Geometry: final body of the model. Coordinates: model frame, mm. A direction names the side the tool comes from. Give positions to 0.01 mm unless a question says otherwise; leave off trailing zeros. Write each loop counter-clockwise with the first axis right and the second up, starting at its lowest first coordinate (ties: lowest second). Pieces come first, ordered by that corner, then holes.
Autodesk Inventor part; units mm, degrees
ref_plane "BODY_N_XY" through (84, 0, 0) normal (0, 0, -1) x (1, 0, 0)
ref_plane "BODY_N_YZ" through (84, 0, 0) normal (1, 0, 0) x (0, -1, 0)
ref_plane "BODY_N_ZX" through (84, 0, 0) normal (0, -1, 0) x (0, 0, -1)
sketch "Sketch_8" plane through (0, 0, 0) normal (0, 0, 1) x (1, 0, 0)
  line L0 (0, 0) -> (-8, 0)
  line L1 (-8, 0) -> (-8, 3.3865)
  line L2 (-8, 3.3865) -> (-7.3865, 4)
  line L3 (-7.3865, 4) -> (0, 4)
  line L4 (0, 4) -> (0, 0)
  line L5 (0, 0) -> (-8, 0)
revolve "Revolution1" add sketch "Sketch_8" angle 360 about axis through (0, 0, 0) along (1, 0, 0)
thread "Thread1"
sketch "Sketch_9" plane through (0, 0, 0) normal (1, 0, 0) x (0, 0, -1)
  line L0 (-6, 3.6056) -> (-6, -3.6056)
  arc A0 (-6, -3.6056) -> (-3.6056, -6) centre (0, 0) ccw
  line L1 (-3.6056, -6) -> (3.6056, -6)
  arc A1 (3.6056, -6) -> (6, -3.6056) centre (0, 0) ccw
  line L2 (6, -3.6056) -> (6, 3.6056)
  arc A2 (6, 3.6056) -> (3.6056, 6) centre (0, 0) ccw
  line L3 (3.6056, 6) -> (-3.6056, 6)
  arc A3 (-3.6056, 6) -> (-6, 3.6056) centre (0, 0) ccw
extrude "Extrusion1" add sketch "Sketch_9" along normal blind 12.5
sketch "Sketch_6" plane through (12.5, 0, 0) normal (1, 0, 0) x (0, 0, -1)
  circle A0 centre (0, 0) radius 5.5
extrude "Extrusion2" add sketch "Sketch_6" along normal blind 54
sketch "Sketch_10" plane through (66.5, 0, 0) normal (1, 0, 0) x (0, 0, -1)
  line L0 (-6, 3.6056) -> (-6, -3.6056)
  arc A0 (-6, -3.6056) -> (-3.6056, -6) centre (0, 0) ccw
  line L1 (-3.6056, -6) -> (3.6056, -6)
  arc A1 (3.6056, -6) -> (6, -3.6056) centre (0, 0) ccw
  line L2 (6, -3.6056) -> (6, 3.6056)
  arc A2 (6, 3.6056) -> (3.6056, 6) centre (0, 0) ccw
  line L3 (3.6056, 6) -> (-3.6056, 6)
  arc A3 (-3.6056, 6) -> (-6, 3.6056) centre (0, 0) ccw
extrude "Extrusion3" add sketch "Sketch_10" along normal blind 22.5
sketch "Sketch7" plane through (0, 0, 0) normal (0, 0, 1) x (1, 0, 0)
  line L0 (8, 6) -> (8, 1)
  line L1 (8, -0.1934) -> (5.933, 1)
  line L2 (5.933, 1) -> (5.933, 5.567)
  line L3 (5.933, 5.567) -> (5.5, 6)
  line L4 (5.5, 6) -> (8, 6)
  line L5 (8, 6) -> (8, -0.1934)
revolve "Revolution2" cut sketch "Sketch7" angle 360 about axis through (8, 6, 0) along (0, 1, 0)
thread "Thread2"
sketch "Sketch_7" plane through (0, 0, 0) normal (0, 0, 1) x (1, 0, 0)
  line L0 (71, 6) -> (71, 1)
  line L1 (71, -0.1934) -> (68.933, 1)
  line L2 (68.933, 1) -> (68.933, 5.567)
  line L3 (68.933, 5.567) -> (68.5, 6)
  line L4 (68.5, 6) -> (71, 6)
  line L5 (71, 6) -> (71, -0.1934)
revolve "Revolution3" cut sketch "Sketch_7" angle 360 about axis through (71, 6, 0) along (0, 1, 0)
thread "Thread3"
sketch "Sketch_16" plane through (0, 0, 0) normal (0, 0, 1) x (1, 0, 0)
  line L0 (47.5, 0) -> (-8, 0)
  line L1 (-8, 0) -> (-8, 2)
  line L2 (-8, 2) -> (12.5, 2)
  line L3 (12.5, 2) -> (12.5, 5)
  line L4 (12.5, 5) -> (47.5, 5)
  line L5 (47.5, 5) -> (47.5, 0)
  line L6 (47.5, 0) -> (-8, 0)
revolve "Revolution4" cut sketch "Sketch_16" angle 360 about axis through (47.5, 0, 0) along (1, 0, 0)
sketch "Sketch_3" plane through (0, 0, 0) normal (0, 1, 0) x (-1, 0, 0)
  line L0 (-76, 1.6) -> (-89, 1.6)
  line L1 (-89, 1.6) -> (-89, -1.6)
  line L2 (-89, -1.6) -> (-76, -1.6)
  line L3 (-76, -1.6) -> (-76, 1.6)
extrude "Extrusion4" cut sketch "Sketch_3" along normal mid plane 12
sketch "Sketch_13" plane through (0, 0, 0) normal (0, 0, 1) x (1, 0, 0)
  circle A0 centre (84, 0) radius 1.65
extrude "Extrusion5" cut sketch "Sketch_13" along normal mid plane 12
ref_plane "BODY_N_XY" through (84, 0, 0) normal (0, 0, -1) x (1, 0, 0)
ref_plane "BODY_N_YZ" through (84, 0, 0) normal (1, 0, 0) x (0, -1, 0)
ref_plane "BODY_N_ZX" through (84, 0, 0) normal (0, -1, 0) x (0, 0, -1)
ref_plane "BODY_PIN_XY" through (84, 0, 0) normal (-1, 0, 0) x (0, 0, -1)
ref_plane "BODY_PIN_YZ" through (84, 0, 0) normal (0, 0, -1) x (0, -1, 0)
ref_plane "BODY_PIN_ZX" through (84, 0, 0) normal (0, -1, 0) x (-1, 0, 0)
ref_plane "NUT2_XY" through (76, 0, 0) normal (1, 0, 0) x (0, 0, -1)
ref_plane "NUT2_YZ" through (76, 0, 0) normal (0, 0, -1) x (0, 1, 0)
ref_plane "NUT2_ZX" through (76, 0, 0) normal (0, 1, 0) x (1, 0, 0)
ref_plane "SW1_XY" through (17, 0, 0) normal (1, 0, 0) x (0, 0, -1)
ref_plane "SW1_YZ" through (17, 0, 0) normal (0, 0, -1) x (0, 1, 0)
ref_plane "SW1_ZX" through (17, 0, 0) normal (0, 1, 0) x (1, 0, 0)
ref_plane "SW2_XY" through (62, 0, 0) normal (-1, 0, 0) x (0, 0, -1)
ref_plane "SW2_YZ" through (62, 0, 0) normal (0, 0, -1) x (0, -1, 0)
ref_plane "SW2_ZX" through (62, 0, 0) normal (0, -1, 0) x (-1, 0, 0)
ref_plane "SW_R1_XY" through (17, -11, 0) normal (1, 0, 0) x (0, 0, -1)
ref_plane "SW_R1_YZ" through (17, -11, 0) normal (0, 0, -1) x (0, 1, 0)
ref_plane "SW_R1_ZX" through (17, -11, 0) normal (0, 1, 0) x (1, 0, 0)
ref_plane "SW_R2_XY" through (62, -11, 0) normal (-1, 0, 0) x (0, 0, -1)
ref_plane "SW_R2_YZ" through (62, -11, 0) normal (0, 0, -1) x (0, -1, 0)
ref_plane "SW_R2_ZX" through (62, -11, 0) normal (0, -1, 0) x (-1, 0, 0)
ref_plane "body_XY" through (0, 0, 0) normal (-1, 0, 0) x (0, 0, -1)
ref_plane "body_YZ" through (0, 0, 0) normal (0, 0, -1) x (0, -1, 0)
ref_plane "body_ZX" through (0, 0, 0) normal (0, -1, 0) x (-1, 0, 0)
properties part number "CJ2D10-30Z(1_0)_BODY"
Item 1: Section C-C, the plane x = 8. Return the cut outline in (y, z), plus the area to 3 significant figures.
Found:
outline: (-6, -3.61) arc R7 ccw to (-3.61, -6) - (3.61, -6) arc R7 ccw to (6, -3.61) - (6, -2.5) - (5.57, -2.07) - (1, -2.07) - (0.85, -1.81) arc R2 cw (long way) to (0.85, 1.81) - (1, 2.07) - (5.57, 2.07) - (6, 2.5) - (6, 3.61) arc R7 ccw to (3.61, 6) - (-3.61, 6) arc R7 ccw to (-6, 3.61) - close
area: 103 mm2
Item 2: Reachability of faces 1 (the face through (66.5, -5, 3)), 2 (the face through (2, -2, 0)), 3 (the face through (76, 0, 0)), 4 (the face through (6, 0, -6)), 5 (the face through (10.065, 3.315, 0.091)) from +Z, -Z, +X, -X, +Y, -Y: full face, straight path, thin tool, end or side. Return the list, or none.
Found:
face 1: none
face 2: -X
face 3: +X, +Y, -Y
face 4: -Z, +X, -X, +Y, -Y
face 5: +Y
Item 3: Line query: L1, parallel to Y at x = -2, z = -0.25; L2, parallel to X at y = -2.75, z = -3.5; L3, parallel to X at y = 0.75, z = -2. Output: solid intervals per line, ascending.
Found:
L1: y = -3.99 to -1.98, 1.98 to 3.99
L2: x = 0 to 12.5, 47.5 to 89
L3: x = -8 to 12.5, 47.5 to 82.53, 85.47 to 89
Item 4: Section B-B, the plane x = 32.5. Return the cut outline in (y, z), plus the area to 3 significant figures.
Found:
outline: circle Ø11 at (0, 0); hole circle Ø10 at (0, 0)
area: 16.5 mm2
Item 5: Section A-A, the plane x = 84. Return the cut outline in (y, z).
Found:
outline: (-6, -3.61) arc R7 ccw to (-3.61, -6) - (-1.65, -6) - (-1.65, -1.6) - (-6, -1.6) - close; (-6, 1.6) - (-1.65, 1.6) - (-1.65, 6) - (-3.61, 6) arc R7 ccw to (-6, 3.61) - close; (1.65, -6) - (3.61, -6) arc R7 ccw to (6, -3.61) - (6, -1.6) - (1.65, -1.6) - close; (1.65, 1.6) - (6, 1.6) - (6, 3.61) arc R7 ccw to (3.61, 6) - (1.65, 6) - close
Item 6: Pull-direction query (Y, two-part tool) for faces 6 (the face through (78, 6, -2)), 7 (the face through (82.35, -0.07, 3.77)), 8 (the face through (77.6, -4.9, -5)); classes: +Y half, -Y half, draft (parallel to the pull), parting line (faces both ways), or undercut.
Found:
face 6: +Y half
face 7: undercut
face 8: -Y half
Item 7: Pin query (flat end, axial travel): pin 1 Ø4.5 at (x, y) = (84, 0) entering from +Z; pin 2 Ø3.5 at (x, z) = (71, 0) entering from +Y; pin 3 Ø3 at (x, z) = (43.5, 4.5) entering from +Y; pin 4 Ø5 at (x, z) = (45, -4.5) entering from +Y. Return the tip coordinate at first contact, or that it passes through.
Found:
pin 1: stops at z = 6
pin 2: stops at y = 0.82
pin 3: stops at y = 4.61
pin 4: stops at y = 5.12
